Input: part model. Units: mm. Frame: model coordinates. Face numbers are marked on the shaded views. Coordinates: 2 decimals unless noted, no trailing zeros. Order: outer loops, then holes, each group sorted by start corner. A loop starts at its lowest first (then second) coordinate and runs counter-clockwise, first axis right, second up. Notation, with made-up numbers: (30.25, 4.25) - (72.25, 4.25) arc R29 ccw to (72.25, 38.25) - close; hole circle Ø1 at (17, 47). An arc over 180 degrees is marked (long way). One line per question, with ' | ' between items. Start each with the question number.
```python
from build123d import *

# Parameters (mm, degrees)
SKETCH1_W           = 12.7
SKETCH1_H           = 12.7
SKETCH1_R           = 2.7
BOSS_EXTRUDE1_DEPTH = 28.275
FILLET2_R           = 1


with BuildPart() as part:
    # Sketch1 → Boss-Extrude1 (new, symmetric)
    with BuildSketch(Plane.XY):
        Rectangle(SKETCH1_W, SKETCH1_H)
        Circle(SKETCH1_R, mode=Mode.SUBTRACT)
    extrude(amount=BOSS_EXTRUDE1_DEPTH, both=True)

    # Fillet2
    fillet2_edges = [part.edges().sort_by_distance(p)[0] for p in [
        (6.35, -6.35, 0),
        (-6.35, -6.35, 0),
        (-6.35, 6.35, 0),
        (6.35, 6.35, 0),
    ]]
    fillet(fillet2_edges, radius=FILLET2_R)


solid = part.part
```
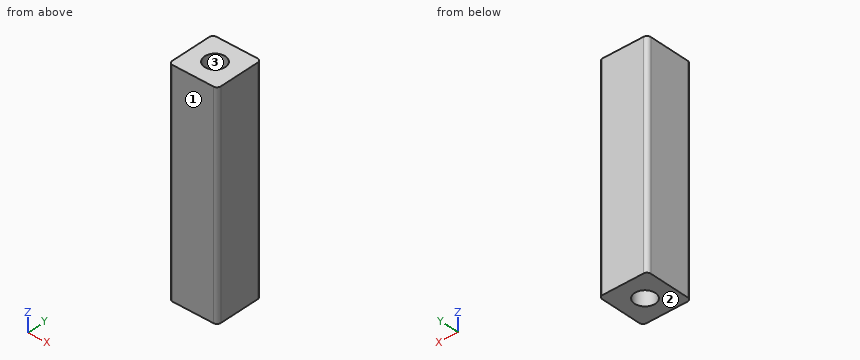
(1) Draft query along Y for the marked faces 1, 2 and 3. Return one class per face: +Y half, -Y half, draft (parallel to the pull), parting line (faces both ways), or undercut.
(2) Section C-C (z = -22). Output: boundary loops of the cut face in (x, y).
(3) Section A-A (y = 0). Output: boundary loops of the cut face in (x, z) (3 decimals), then the cut area to 3 significant figures.
(4) Material intervals for line 1 along Y through (x, z) = (0, 6); line 2 along X through (y, z) = (-0.5, 10.5); line 3 along Y through (x, z) = (1.5, -1.5) (3 decimals), sorted ascending. Write a range as from..to.
(5) Pin query (flat end, axial travel): pin 1 (4 mm diameter, centred on x = -2, y = -1, fed in from -Z) (3 decimals); pin 2 (3 mm diameter, centred on x = -0.5, y = 1, fed in from -Z). Return the tip coordinate at first contact, or that it passes through.
Worked answers:
1) face 1: -Y half | face 2: draft | face 3: undercut
2) outline: (-6.35, -5.35) arc R1 ccw to (-5.35, -6.35) - (5.35, -6.35) arc R1 ccw to (6.35, -5.35) - (6.35, 5.35) arc R1 ccw to (5.35, 6.35) - (-5.35, 6.35) arc R1 ccw to (-6.35, 5.35) - close; hole circle Ø5.4 at (0, 0)
3) outline: (-6.35, -28.275) - (-2.7, -28.275) - (-2.7, 28.275) - (-6.35, 28.275) - close; (2.7, -28.275) - (6.35, -28.275) - (6.35, 28.275) - (2.7, 28.275) - close | area: 413 mm²
4) line 1: y = -6.35..-2.7, 2.7..6.35 | line 2: x = -6.35..-2.65, 2.65..6.35 | line 3: y = -6.35..-2.245, 2.245..6.35
5) pin 1: stops at z = -28.275 | pin 2: passes through
